from build123d import *

# Parameters (mm, degrees)
SKETCH1_R           = 5.2
SKETCH1_R_2         = 3.2
BOSS_EXTRUDE1_DEPTH = 7
SKETCH2_R           = 9.525
BOSS_EXTRUDE2_DEPTH = 10
BOSS_EXTRUDE3_START = 0.8
BOSS_EXTRUDE3_DEPTH = 0.8


with BuildPart() as part:
    # Sketch1 → Boss-Extrude1 (new body)
    with BuildSketch(Plane(origin=(0, 0, 0), x_dir=(1, 0, 0), z_dir=(0, 1, 0))):
        with Locations(Location((0, 0, 0), (0, 0, 270))):
            Circle(SKETCH1_R)
        with Locations(Location((0, 0, 0), (0, 0, 270))):
            Circle(SKETCH1_R_2, mode=Mode.SUBTRACT)
    extrude(amount=BOSS_EXTRUDE1_DEPTH)

    # Sketch2 → Boss-Extrude2 (add)
    with BuildSketch(Plane(origin=(0, 7, 0), x_dir=(1, 0, 0), z_dir=(0, 1, 0))):
        with Locations(Location((0, 0, 0), (0, 0, 270))):
            Circle(SKETCH2_R)
    extrude(amount=BOSS_EXTRUDE2_DEPTH)

    # Sketch3 → Boss-Extrude3 (add)
    with BuildSketch(Plane.XZ.offset(-7).offset(BOSS_EXTRUDE3_START)):
        with BuildLine():
            Line((3.122498999, 0.7), (-3.122498999, 0.7))
            ThreePointArc((-3.122498999, 0.7), (-3.180565736, 0.352138611), (-3.2, 0))
            ThreePointArc((-3.2, 0), (-3.180565736, -0.352138611), (-3.122498999, -0.7))
            Line((-3.122498999, -0.7), (3.122498999, -0.7))
            ThreePointArc((3.122498999, -0.7), (3.180565736, -0.352138611), (3.2, 0))
            ThreePointArc((3.2, 0), (3.180565736, 0.352138611), (3.122498999, 0.7))
        make_face()
    extrude(amount=-BOSS_EXTRUDE3_DEPTH)


solid = part.part
Verification items for the finished model (mm, model axes). A direction names the side the tool comes from. Round coordinates to 2 decimals unless told otherwise and drop trailing zeros. Loops run counter-clockwise (first coordinate to the right, second up) from the corner with the lowest first, then second, coordinate; pieces in that order, holes last. Notation, with made-up numbers: (74.5, 86.5) - (86.5, 86.5) arc R20 cw to (86.5, 103.5) - close; hole circle Ø2 at (-29, -24). An arc over 180 degrees is marked (long way). Write item = value, one per line.
Q1. Sectioned sample at A-A on z = 0. Record the boundary of the cut face in (x, y) (3 decimals).
Here are the results:
outline = (-9.525, 7) - (-5.2, 7) - (-5.2, 0) - (-3.2, 0) - (-3.2, 6.2) - (3.2, 6.2) - (3.2, 0) - (5.2, 0) - (5.2, 7) - (9.525, 7) - (9.525, 17) - (-9.525, 17) - close
Q2. Sectioned sample at D-D on y = 8. Record the boundary of the cut face in (x, z) (3 decimals), plus the area to 3 significant figures.
Here are the results:
outline = circle Ø19.05 at (0, 0)
area = 285 mm^2
Q3. Tool access check on faces 1 (the flat face through (0, 17, 0)), 2 (the flat face through (0, 7, -2)). Record the directions out of +Z, -Z, +X, -X, +Y, -Y that give a thin tool (end or side, any length) a straight path to the whole face; none if there is none.
Here are the results:
face_1 = +Z, -Z, +X, -X, +Y
face_2 = -Y
Q4. Depth check by flat-ended pin: pin 1 (1 mm diameter, centred on y = 7.5, z = -4.5, fed in from -X); pin 2 (0.8 mm diameter, centred on x = -1.5, z = 2, fed in from -Y); pin 3 (0.7 mm diameter, centred on x = 1.5, z = 0, fed in from -Y); pin 4 (10 mm diameter, centred on x = 0, z = 0, fed in from -Y). Enter the tip coordinate at first touch or a pass-through.
Here are the results:
pin_1 = -8.64
pin_2 = 7
pin_3 = 6.2
pin_4 = 0
Q5. Sectioned sample at B-B on x = 0. Record the boundary of the cut face in (y, z) (3 decimals).
Here are the results:
outline = (0, -5.2) - (7, -5.2) - (7, -9.525) - (17, -9.525) - (17, 9.525) - (7, 9.525) - (7, 5.2) - (0, 5.2) - (0, 3.2) - (7, 3.2) - (7, 0.7) - (6.2, 0.7) - (6.2, -0.7) - (7, -0.7) - (7, -3.2) - (0, -3.2) - close
Q6. Material ranges on L1, parallel to X at y = 2, z = 0; L2, parallel to Z at x = -0.25, y = 12.25; L3, parallel to Y at x = -8, z = 4.75, recorded low to high.
Here are the results:
L1 = -5.2 to -3.2, 3.2 to 5.2
L2 = -9.52 to 9.52
L3 = 7 to 17
Q7. Sectioned sample at C-C on y = 2.5. Record the boundary of the cut face in (x, z), plus the area to 3 significant figures.
Here are the results:
outline = circle Ø10.4 at (0, 0); hole circle Ø6.4 at (0, 0)
area = 52.8 mm^2
Q8. Mould release check, pull along X, two halves, no side actions. Record for faces 3 (the cylindrical face through (1.56, 3.45, 4.96)), 4 (the flat face through (0, 6.2, 0)), 5 (the flat face through (-4, 7, 4)): +X half, -X half, draft (parallel to the pull), parting line (faces both ways), or undercut.
Here are the results:
face_3 = parting line
face_4 = undercut
face_5 = draft
